For this review, take the finished solid that the model builds, in its own axes (mm). A direction names the side the tool comes from. Coordinates: 2 decimals unless noted, no trailing zeros. Write each loop counter-clockwise with the first axis right and the second up, starting at its lowest first coordinate (ties: lowest second). Pieces come first, ordered by that corner, then holes. Notation, with made-up numbers: (-37, 31) - (-13, 31) arc R16 cw to (-13, 58) - close; hole circle Ø1 at (30, 62). An arc over 180 degrees is marked (long way). Use one line per item in the form item = value. Start each with the question number.
1) We need section B-B (x = -11). Give the boundary of the cut face in (y, z), plus the area to 3 significant figures.
2) We need section A-A (z = 0.5). Give the boundary of the cut face in (x, y).
3) We need section D-D (x = -2.75). Give the boundary of the cut face in (y, z), plus the area to 3 significant figures.
4) Tool access review of faces 1 (the flat face through (-7.353, 8, 0)), 2 (the cylindrical face through (9.06, 0.81, -4.44)), 3 (the flat face through (7.353, 8, 0)): name each direction out of +Z, -Z, +X, -X, +Y, -Y from which nothing blocks a thin tool from reaching the whole face with its end or side.
5) Mouldability with a two-part tool opening along Z and no side actions: class faces 4 (the cylindrical face through (-11.844, 0.811, -4.444)), 5 (the flat face through (0, 8, -4.254)), 6 (the flat face through (0, 8, 4.254)), 7 (the flat face through (13.348, 1, 0)) as pulls with the +Z half, pulls with the -Z half, needs draft (parallel to the pull), parting line crosses it, or undercut.
6) For L1, parallel to X at y = 7.25, z = -2.25; L2, parallel to Y at x = 10, z = 0; L3, parallel to Z at x = 6.75, y = 8.25, list the stretches that pass through material, from the lowest coordinate up. Write a range as from..to.
7) Insertion check: P1, Ø6, axis at x = 3, y = 10, coming from the +Z side; P2, Ø5.5, axis at x = -10.45, z = -3.56, coming from the +Y side; P3, Ø1, axis at y = 2.5, z = -4.5, coming from the +X side. Each pin has a flat end and moves straight along its axis. Give the tip position at first contact, or say it passes through.
8) We need section C-C (z = 3.5). Give the boundary of the cut face in (x, y), plus the area to 3 significant figures.
Autodesk Inventor part; units mm, degrees
ref_plane "YZ Plane" through (0, 0, 0) normal (1, 0, 0) x (0, 1, 0)
ref_plane "XZ Plane" through (0, 0, 0) normal (0, 1, 0) x (-1, 0, 0)
ref_plane "XY Plane" through (0, 0, 0) normal (0, 0, 1) x (1, 0, 0)
sketch "Sketch5" plane through (0, 0, 0) normal (0, 1, 0) x (-1, 0, 0)
  line L0 (13.3477, 6.4516) -> (-13.3477, 6.4516)
  line L1 (-13.3477, 6.4516) -> (-13.3477, -6.4516)
  line L2 (-13.3477, -6.4516) -> (13.3477, -6.4516)
  line L3 (13.3477, -6.4516) -> (13.3477, 6.4516)
  line L4 (13.3477, 6.4516) -> (-13.3477, -6.4516) construction
  line L5 (-13.3477, 6.4516) -> (13.3477, -6.4516) construction
  point P0 (0, 0)
  dimension "d25" = 26.6954
  dimension "d26" = 12.9032
extrude "Extrusion3" add sketch "Sketch5" along normal blind 1.6002
sketch "Sketch6" plane through (0, 1.6002, 0) normal (0, 1, 0) x (1, 0, 0)
  line L0 (-7.3533, -4.2545) -> (7.3533, -4.2545)
  line L1 (7.3533, -4.2545) -> (7.3533, 4.2545)
  line L2 (7.3533, 4.2545) -> (-7.3533, 4.2545)
  line L3 (-7.3533, 4.2545) -> (-7.3533, -4.2545)
  line L4 (-7.3533, -4.2545) -> (7.3533, 4.2545) construction
  line L5 (7.3533, -4.2545) -> (-7.3533, 4.2545) construction
  point P0 (0, 0)
  dimension "d29" = 14.7066
  dimension "d30" = 8.509
extrude "Extrusion4" add sketch "Sketch6" along normal blind 13.589
sketch "Sketch7" plane through (0, 0, 0) normal (0, -1, 0) x (1, 0, 0)
  line L0 (-10.4521, -3.556) -> (10.4521, -3.556) construction
  line L1 (10.4521, -3.556) -> (10.4521, 3.556) construction
  line L2 (10.4521, 3.556) -> (-10.4521, 3.556) construction
  line L3 (-10.4521, 3.556) -> (-10.4521, -3.556) construction
  line L4 (-10.4521, -3.556) -> (10.4521, 3.556) construction
  line L5 (10.4521, -3.556) -> (-10.4521, 3.556) construction
  point P0 (0, 0)
  dimension "d33" = 20.9042
  dimension "d34" = 7.112
hole "Hole3" at (-10.4521, 0, 3.556) at (10.4521, 0, 3.556) at (10.4521, 0, -3.556) at (-10.4521, 0, -3.556) direction (0, 1, 0) diameter 3.302 end through all
equation "\"d25\" = CanBaseWidth"
equation "\"d26\" = CanBaseLength"
equation "\"d27\" = pcBoardDepth"
equation "\"d29\" = connectorWidth"
equation "\"d30\" = connectorLength"
equation "\"d31\" = connectorHeight"
equation "\"d33\" = HoleWidth"
equation "\"d34\" = HoleLength"
equation "\"CanBaseWidth\" = 26.6954"
equation "\"CanBaseLength\" = 12.9032"
equation "\"HoleWidth\" = 20.9042"
equation "\"HoleLength\" = 7.112"
equation "\"BaseOffset\" = 5.08"
equation "\"PartWidth\" = CanBaseWidth + 2 * BaseOffset"
equation "\"PartLength\" = CanBaseLength + 2 * BaseOffset"
equation "\"boardGap\" = 0.508"
equation "\"boltHeadHeight\" = 3.175"
equation "\"boltHeadDiam\" = 5.08"
equation "\"pcBoardDepth\" = 1.6002"
equation "\"connectorWidth\" = 14.7066"
equation "\"connectorLength\" = 8.509"
equation "\"connectorHeight\" = 13.589"
properties part number "canConnectorModel"
Determined:
q1.outline = (0, -6.45) - (1.6, -6.45) - (1.6, -5.11) - (0, -5.11) - close; (0, -2) - (1.6, -2) - (1.6, 2) - (0, 2) - close; (0, 5.11) - (1.6, 5.11) - (1.6, 6.45) - (0, 6.45) - close
q1.area = 10.7 mm²
q2.outline = (-13.35, 0) - (13.35, 0) - (13.35, 1.6) - (7.35, 1.6) - (7.35, 15.19) - (-7.35, 15.19) - (-7.35, 1.6) - (-13.35, 1.6) - close
q3.outline = (0, -6.45) - (1.6, -6.45) - (1.6, -4.25) - (15.19, -4.25) - (15.19, 4.25) - (1.6, 4.25) - (1.6, 6.45) - (0, 6.45) - close
q3.area = 136 mm²
q4.face_1 = +Z, -Z, -X, +Y
q4.face_2 = +Y, -Y
q4.face_3 = +Z, -Z, +X, +Y
q5.face_4 = undercut
q5.face_5 = pulls with the -Z half
q5.face_6 = pulls with the +Z half
q5.face_7 = needs draft
q6.L1 = -7.35..7.35
q6.L2 = 0..1.6
q6.L3 = -4.25..4.25
q7.P1 = 4.25
q7.P2 = 1.6
q7.P3 = 7.35
q8.outline = (-13.35, 0) - (-12.1, 0) - (-12.1, 1.6) - (-13.35, 1.6) - close; (-8.8, 0) - (8.8, 0) - (8.8, 1.6) - (7.35, 1.6) - (7.35, 15.19) - (-7.35, 15.19) - (-7.35, 1.6) - (-8.8, 1.6) - close; (12.1, 0) - (13.35, 0) - (13.35, 1.6) - (12.1, 1.6) - close
q8.area = 232 mm²
